from build123d import *

# Parameters (mm, degrees)
F1_DEPTH = 50
F2_W     = 20
F2_H     = 5
F3_DEPTH = 15


with BuildPart() as f1:
    # F0 (on Right) → F1 (new body)
    with BuildSketch(Plane.YZ):
        Polygon((0, 40), (-20, 40), (-40, 15), (-40, 0), (0, 0), align=None)
    extrude(amount=-F1_DEPTH)

    # F2 (on face) → F3 (cut)
    with BuildSketch(Plane.XZ.offset(40)):
        with Locations((-25, 2.5)):
            Rectangle(F2_W, F2_H)
    extrude(amount=-F3_DEPTH, mode=Mode.SUBTRACT)


solid = f1.part
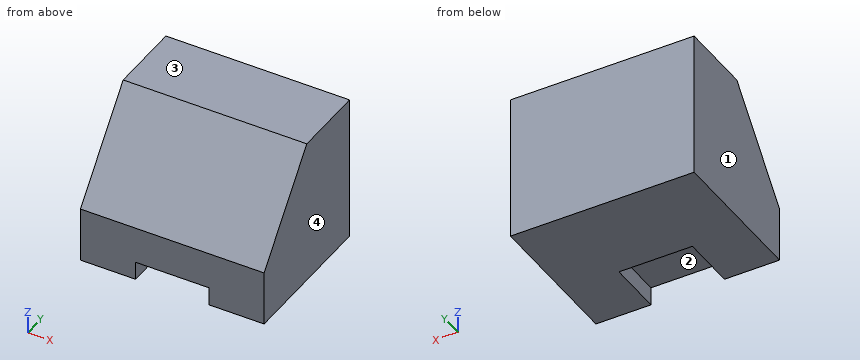
Source: CAD feature listing. Evaluate the final solid. Frame: model axes, mm. Face numbers are marked on the shaded views. Give positions to 0.01 mm unless a question says otherwise; leave off trailing zeros. Write each loop counter-clockwise with the first axis right and the second up, starting at its lowest first coordinate (ties: lowest second). Pieces come first, ordered by that corner, then holes. Notation, with made-up numbers: (-19.75, 8.5) - (13.25, 8.5) arc R22 cw to (13.25, 19.5) - close; hole circle Ø9 at (80, 31.5). An arc over 180 degrees is marked (long way). Write item = value, one per line. Start each with the question number.
Q1. Cut plane A-A, the plane y = -28. Return loops of the section in (x, z), then the cut area to 3 significant figures.
Q2. Cut plane D-D, the plane y = -23. Return loops of the section in (x, z), then the cut area to 3 significant figures.
Q3. Material intervals for probe 1 along Z at (x, y) = (-24, -33); probe 2 along Y at (x, z) = (-44, 21); probe 3 along Z at (x, y) = (-43.5, -36.5) (3 decimals), sorted ascending.
Q4. Cut plane B-B, the plane x = -40. Return loops of the section in (y, z).
Q5. Pin query (flat end, axial travel): pin 1 Ø5 at (x, z) = (-39.5, 33) entering from -Y; pin 2 Ø4 at (x, z) = (-40, 19.5) entering from -Y. Return the tip coordinate at first contact, or that it passes through.
Q6. Cut plane C-C, the plane z = 3. Return loops of the section in (x, y), then the cut area to 3 significant figures.
Q7. Draft query along X for the marked faces 1, 2, 3 and 4. Return one class per face: +X half, -X half, draft (parallel to the pull), parting line (faces both ways), or undercut.
Computed values:
q1.outline = (-50, 0) - (-35, 0) - (-35, 5) - (-15, 5) - (-15, 0) - (0, 0) - (0, 30) - (-50, 30) - close
q1.area = 1,400 mm²
q2.outline = (-50, 0) - (0, 0) - (0, 36.25) - (-50, 36.25) - close
q2.area = 1,810 mm²
q3.probe_1 = 5 to 23.75
q3.probe_2 = -35.2 to 0
q3.probe_3 = 0 to 19.375
q4.outline = (-40, 0) - (0, 0) - (0, 40) - (-20, 40) - (-40, 15) - close
q5.pin_1 = -27.6
q5.pin_2 = -38
q6.outline = (-50, -40) - (-35, -40) - (-35, -25) - (-15, -25) - (-15, -40) - (0, -40) - (0, 0) - (-50, 0) - close
q6.area = 1,700 mm²
q7.face_1 = -X half
q7.face_2 = undercut
q7.face_3 = draft
q7.face_4 = +X half
